```python
from build123d import *

# Parameters (mm, degrees)
SKETCH1_R           = 4
BOSS_EXTRUDE1_DEPTH = 32
SKETCH4_R           = 5.5
BOSS_EXTRUDE3_DEPTH = 1
BOSS_EXTRUDE4_DEPTH = 1
SKETCH6_W           = 5
SKETCH6_H           = 8
CUT_EXTRUDE2_DEPTH  = 7.5


with BuildPart() as part:
    # Sketch1 → Boss-Extrude1 (new body)
    with BuildSketch(Plane(origin=(0, 0, 0), x_dir=(1, 0, 0), z_dir=(0, 1, 0))):
        with Locations(Location((0, 0, 0), (0, 0, 270))):
            Circle(SKETCH1_R)
    extrude(amount=BOSS_EXTRUDE1_DEPTH)

    # Sketch4 → Boss-Extrude3 (add)
    with BuildSketch(Plane.XZ):
        with Locations(Location((0, 0, 0), (0, 0, 270))):
            Circle(SKETCH4_R)
    extrude(amount=BOSS_EXTRUDE3_DEPTH)

    # Sketch5 → Boss-Extrude4 (add)
    with BuildSketch(Plane(origin=(0, 31, 0), x_dir=(1, 0, 0), z_dir=(0, 1, 0))):
        with BuildLine():
            Line((-3.75, -3.142053469), (3.75, -3.142053469))
            ThreePointArc((3.75, -3.142053469), (4.892340953, 0), (3.75, 3.142053469))
            Line((3.75, 3.142053469), (-3.75, 3.142053469))
            ThreePointArc((-3.75, 3.142053469), (-4.892340953, 0), (-3.75, -3.142053469))
        make_face()
    extrude(amount=BOSS_EXTRUDE4_DEPTH)

    # Sketch6 → Cut-Extrude2 (cut)
    with BuildSketch(Plane(origin=(0, 32, 0), x_dir=(1, 0, 0), z_dir=(0, 1, 0))):
        Rectangle(SKETCH6_W, SKETCH6_H)
    extrude(amount=-CUT_EXTRUDE2_DEPTH, mode=Mode.SUBTRACT)

    # Sketch8 → Cut-Revolve1 (revolve, cut)
    with BuildSketch(Plane.XY, mode=Mode.PRIVATE) as cut_revolve1_sk:
        Polygon((4.892340953, 31), (4, 32), (4.892340953, 32), align=None)
    revolve(cut_revolve1_sk.sketch.rotate(Axis((0, 0, 0), (0, 1, 0)), 90), axis=Axis((0, 0, 0), (0, 1, 0)), mode=Mode.SUBTRACT)


solid = part.part
```
Part model, mm, in its own coordinate system. A direction names the side the tool comes from. Coordinates: 2 decimals unless noted, no trailing zeros. Write each loop counter-clockwise with the first axis right and the second up, starting at its lowest first coordinate (ties: lowest second). Pieces come first, ordered by that corner, then holes.
Item 1: Slice it at B-B (x = 0). Write the cut outline in (y, z).
Item 2: Slice it at C-C (y = 21.5). Write the cut outline in (x, z), and give its area (3 significant figures).
Item 3: Mould opens along X. For faces 6 (the face through (-2.5, 28, 0)), 7 (the face through (4.24, 31.73, 0.05)), 8 (the face through (-3, 32, 0)) say: released by +X, released by -X, zero draft, split by the parting line, or undercut.
Item 4: Which spindle directions (+Z, -Z, +X, -X, +Y, -Y) get a long thin tool onto all of the face, cutting with end or side? Do faces 1 (the face through (3.966, 15.283, -0.521)), 2 (the face through (4.2, 31, 0)), 3 (the face through (3, 31.4, 3.142)), 4 (the face through (-4.2, 31, 0)), 5 (the face through (2.5, 28, 0)). Say none if no direction does.
Item 5: Slice it at D-D (z = 4.75). Write the cut outline in (x, y), and give its area (3 significant figures).
Item 6: Pin check, flat tips, straight feed: pin 1 (5 mm diameter, centred on y = 3, z = -1, fed in from +X); pin 2 (1.9 mm diameter, centred on y = 28.5, z = 0, fed in from -X); pin 3 (2 mm diameter, centred on x = 3, y = 26.5, fed in from +Z). Stop position of each tip, or through.
Item 7: Slice it at A-A (z = 0). Write the cut outline in (x, y).
Item 8: Probe line 1 (Y direction, x = -1.5, z = -0.5); line 2 (Z direction, x = 0.25, y = 24). List the from-to ranges inside material, lowest first.
Results found:
1. outline: (-1, -5.5) - (0, -5.5) - (0, -4) - (24.5, -4) - (24.5, 4) - (0, 4) - (0, 5.5) - (-1, 5.5) - close
2. outline: circle Ø8 at (0, 0)
2. area: 50.3 mm2
3. face 6: undercut
3. face 7: released by +X
3. face 8: zero draft
4. face 1: none
4. face 2: +X
4. face 3: +Z, +X, -X, +Y
4. face 4: -X
4. face 5: +Z, -Z, +Y
5. outline: (-2.77, -1) - (2.77, -1) - (2.77, 0) - (-2.77, 0) - close
5. area: 5.55 mm2
6. pin 1: stops at x = 4
6. pin 2: stops at x = -4
6. pin 3: stops at z = 3.12
7. outline: (-5.5, -1) - (5.5, -1) - (5.5, 0) - (4, 0) - (4, 31) - (4.89, 31) - (4, 32) - (2.5, 32) - (2.5, 24.5) - (-2.5, 24.5) - (-2.5, 32) - (-4, 32) - (-4.89, 31) - (-4, 31) - (-4, 0) - (-5.5, 0) - close
8. line 1: y = -1 to 24.5
8. line 2: z = -3.99 to 3.99
